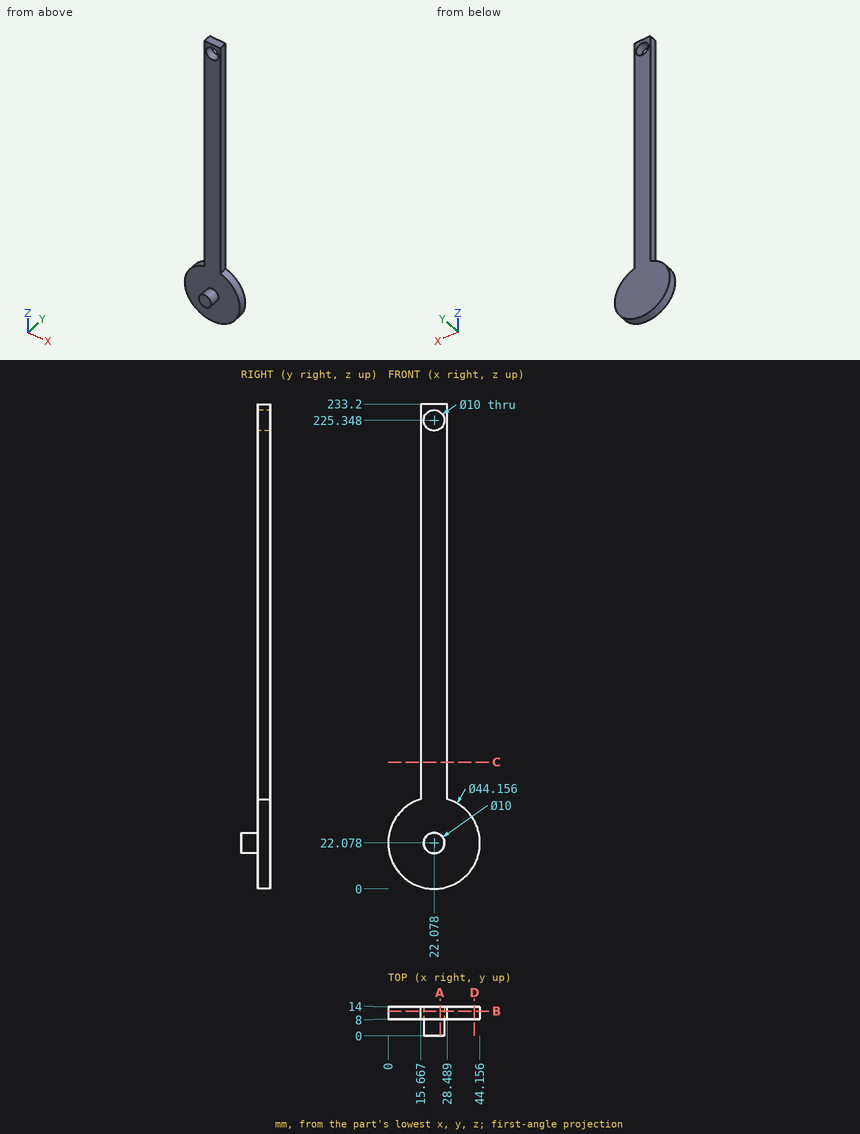
The figure shows three views and two pictorial views of one solid part (mm, origin at its lowest corner). Answer the questions. Give positions to 0.01 mm unless a question says otherwise; leave off trailing zeros. Order: outer loops, then holes, each group sorted by start corner. A loop starts at its lowest first (then second) coordinate and runs counter-clockwise, first axis right, second up. Notation, with made-up numbers: (81.5, -19) -> (118.5, -19) arc R23 cw to (118.5, 19) -> close; hole circle Ø2 at (65, 18.5). An arc over 180 degrees is marked (long way). Answer as CSV lines item,"result". Start each with the question number.
Q1. A cutting plane is placed at B-B (y = 12). Determine the outline of the cut face in (x, z) (1 decimal), then the cut area to 3 significant figures.
Q2. A cutting plane is placed at A-A (x = 25). Determine the outline of the cut face in (y, z) (1 decimal).
Q3. Given pin 1 (8 mm diameter, centred on x = 33, z = 128.5, fed in from +Y); pin 2 (3 mm diameter, centred on x = 24, z = 145.5, fed in from -Y); pin 3 (1 mm diameter, centred on y = 12, z = 156, fed in from +X); pin 4 (3 mm diameter, centred on x = 18.5, y = 3.5, fed in from +Z), each flat-ended and moving along its own axis, determine where each tip first touches the part or whether it passes through.
Q4. A cutting plane is placed at C-C (z = 61). Determine the outline of the cut face in (x, y).
Q5. Find the intervals of material crossed by L1, parallel to X at y = 13, z = 198.5; L2, parallel to Z at x = 17.5, y = 8.75; L3, parallel to Y at x = 35.5, z = 21.5, in increasing order.
Q6. A cutting plane is placed at D-D (x = 41.5). Determine the outline of the cut face in (y, z), then the cut area to 3 significant figures.
Results found:
1,outline,"(15.7, 43.2) arc R22.1 ccw (long way) to (28.5, 43.2) -> (28.5, 233.2) -> (15.7, 233.2) -> close; hole circle Ø10 at (22.1, 225.3)"
1,area,"3,880 mm2"
2,outline,"(0, 18) -> (8, 18) -> (8, 0.2) -> (14, 0.2) -> (14, 221.3) -> (8, 221.3) -> (8, 26.1) -> (0, 26.1) -> close; (8, 229.4) -> (14, 229.4) -> (14, 233.2) -> (8, 233.2) -> close"
3,pin 1,"through"
3,pin 2,"y = 8"
3,pin 3,"x = 28.49"
3,pin 4,"z = 26.63"
4,outline,"(15.67, 8) -> (28.49, 8) -> (28.49, 14) -> (15.67, 14) -> close"
5,L1,"15.67 to 28.49"
5,L2,"0.48 to 223.34, 227.36 to 233.2"
5,L3,"8 to 14"
6,outline,"(8, 11.58) -> (14, 11.58) -> (14, 32.58) -> (8, 32.58) -> close"
6,area,"126 mm2"
